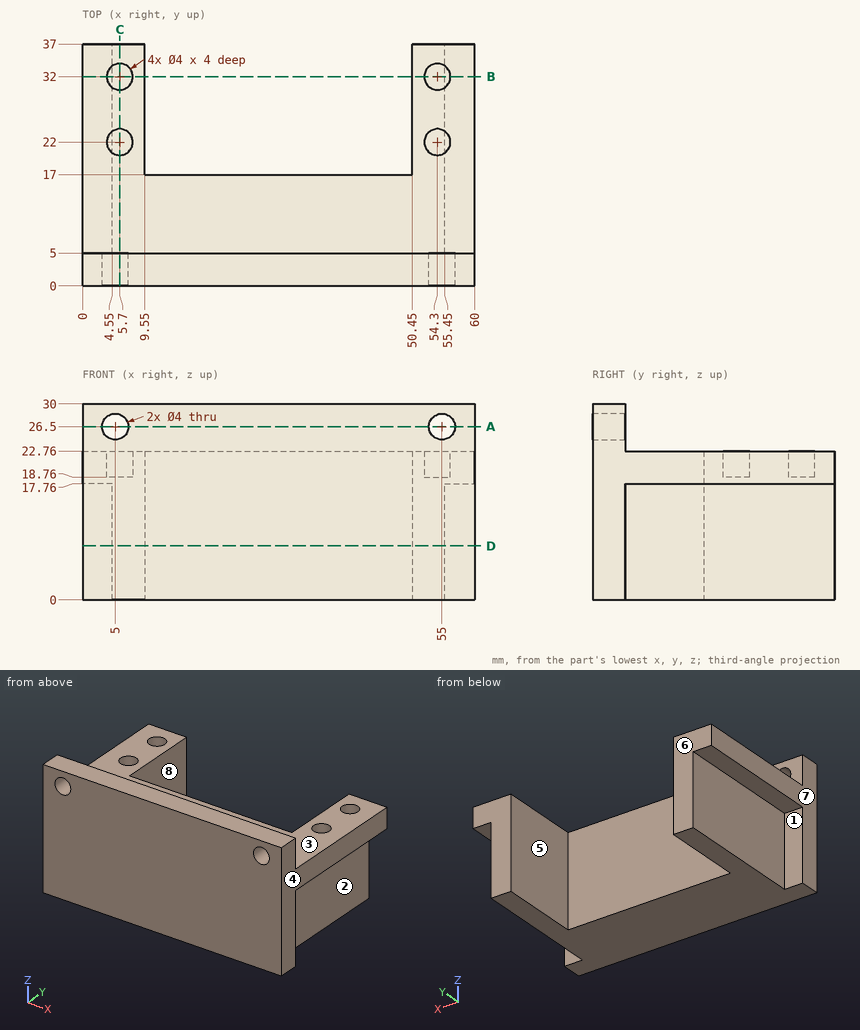
Input: dimensioned drawing with shaded views. Units: mm. Origin: part minimum x, y, z. A direction names the side the tool comes from. Give positions to 0.01 mm unless a question says otherwise; leave off trailing zeros. Write each loop counter-clockwise with the first axis right and the second up, starting at its lowest first coordinate (ties: lowest second). Pieces come first, ordered by that corner, then holes. Notation, with made-up numbers: M -30,29 L 12,29 A12 ccw 12,39 Z; hole C -11,56 d2. An arc over 180 degrees is marked long. Return JSON: item names as keys, results as strings. Group by question number.
1) Cut plane A-A, the plane z = 26.5. Output: boundary loops of the cut face in (x, y), plus the area to 3 significant figures.
2) Pull-direction query (X, two-part tool) for the marked faces 6, 7 and 8; classes: pulls with the +X half, pulls with the -X half, needs draft (parallel to the pull), parting line crosses it, or undercut.
3) Cut plane D-D, the plane z = 8.25. Output: boundary loops of the cut face in (x, y), plus the area to 3 significant figures.
4) Material intervals for line 1 along Y through (x, z) = (5.7, 19.95); line 2 along X through (y, z) = (1.25, 26.5); line 3 along X through (y, z) = (19.5, 1.5), sorted ascending. Write a range as [from, to].
5) Pin query (flat end, axial travel): P1, Ø1.2, axis at x = 54.5, y = 31.5, coming from the +Z side; P2, Ø3, axis at y = 16, z = 10, coming from the -X side; P3, Ø3.5, axis at x = 2, z = 9, coming from the +Y side; P4, Ø3.5, axis at x = 5, z = 26.5, coming from the -Y side. Return the tip coordinate at first contact, or that it passes through.
6) Cut plane B-B, the plane y = 32. Output: boundary loops of the cut face in (x, z), plus the area to 3 significant figures.
7) Cut plane C-C, the plane x = 5.7. Output: boundary loops of the cut face in (y, z), plus the area to 3 significant figures.
8) Set-up query: the marked faces 1, 2, 3, 4 and 5. Return all of +Z, -Z, +X, -X, +Y, -Y with unobstructed straight access to the full face (end or side cutting, diameter ignored); none if empty.
Recorded:
{
 "1": {"outline": "M 0,0 L 3,0 L 3,5 L 0,5 Z; M 7,0 L 53,0 L 53,5 L 7,5 Z; M 57,0 L 60,0 L 60,5 L 57,5 Z", "area": "260 mm²"},
 "2": {"face 6": "needs draft", "face 7": "pulls with the -X half", "face 8": "undercut"},
 "3": {"outline": "M 0,0 L 60,0 L 60,5 L 55.45,5 L 55.45,37 L 50.45,37 L 50.45,17 L 9.55,17 L 9.55,37 L 4.55,37 L 4.55,5 L 0,5 Z", "area": "1,110 mm²"},
 "4": {"line 1": "y = [0, 20], [24, 30], [34, 37]", "line 2": "x = [0, 3], [7, 53], [57, 60]", "line 3": "x = [4.55, 9.55], [50.45, 55.45]"},
 "5": {"P1": "stops at z = 18.76", "P2": "stops at x = 4.55", "P3": "stops at y = 5", "P4": "passes through"},
 "6": {"outline": "M 0,17.76 L 4.55,17.76 L 4.55,0 L 9.55,0 L 9.55,22.76 L 7.7,22.76 L 7.7,18.76 L 3.7,18.76 L 3.7,22.76 L 0,22.76 Z; M 50.45,0 L 55.45,0 L 55.45,17.76 L 60,17.76 L 60,22.76 L 56.3,22.76 L 56.3,18.76 L 52.3,18.76 L 52.3,22.76 L 50.45,22.76 Z", "area": "241 mm²"},
 "7": {"outline": "M 0,0 L 37,0 L 37,22.76 L 34,22.76 L 34,18.76 L 30,18.76 L 30,22.76 L 24,22.76 L 24,18.76 L 20,18.76 L 20,22.76 L 5,22.76 L 5,24.63 L 0,24.63 Z; M 0,28.37 L 5,28.37 L 5,30 L 0,30 Z", "area": "828 mm²"},
 "8": {"face 1": "-Z, -X, +Y", "face 2": "-Z, +X, +Y", "face 3": "+Z, +X, -X, +Y", "face 4": "+Z, -Z, +X, +Y, -Y", "face 5": "+Z, -Z, +Y"}
}
